from build123d import *

# Parameters (mm, degrees)
SKETCH1_W           = 49.022
SKETCH1_H           = 96.52
BOSS_EXTRUDE1_DEPTH = 7.62
SKETCH2_R           = 1.905
CUT_EXTRUDE1_DEPTH  = 55.661514075
SKETCH3_R           = 7.9375
CUT_EXTRUDE2_DEPTH  = 55.661514075
FILLET1_R           = 5.08
FILLET2_R           = 5.08
CUT_EXTRUDE3_DEPTH  = 55.661514075
SKETCH5_R           = 7.9375
SKETCH5_R_2         = 2.54
CUT_EXTRUDE4_DEPTH  = 55.661514075


with BuildPart() as part:
    # Sketch1 → Boss-Extrude1 (new body)
    with BuildSketch(Plane(origin=(0, 0, 0), x_dir=(1, 0, 0), z_dir=(0, 1, 0))):
        Rectangle(SKETCH1_W, SKETCH1_H)
    extrude(amount=BOSS_EXTRUDE1_DEPTH)

    # Sketch2 → Cut-Extrude1 (cut, through all)
    with BuildSketch(Plane(origin=(0, 7.62, 0), x_dir=(1, 0, 0), z_dir=(0, 1, 0))):
        with Locations(Location((-16.891, -44.45, 0), (0, 0, 270))):
            Circle(SKETCH2_R)
        with Locations(Location((-7.62, -44.45, 0), (0, 0, 270))):
            Circle(SKETCH2_R)
        with Locations(Location((7.62, -44.45, 0), (0, 0, 270))):
            Circle(SKETCH2_R)
        with Locations(Location((16.891, -44.45, 0), (0, 0, 270))):
            Circle(SKETCH2_R)
    extrude(amount=-CUT_EXTRUDE1_DEPTH, mode=Mode.SUBTRACT)

    # Sketch3 → Cut-Extrude2 (cut, through all)
    with BuildSketch(Plane(origin=(0, 7.62, 0), x_dir=(1, 0, 0), z_dir=(0, 1, 0))):
        with Locations(Location((0, 35.052, 0), (0, 0, 270))):
            Circle(SKETCH3_R)
    extrude(amount=-CUT_EXTRUDE2_DEPTH, mode=Mode.SUBTRACT)

    # Fillet1
    fillet1_edges = [part.edges().sort_by_distance(p)[0] for p in [
        (-24.511, 3.81, -48.26),
        (24.511, 3.81, -48.26),
    ]]
    fillet(fillet1_edges, radius=FILLET1_R)

    # Fillet2
    fillet2_edges = [part.edges().sort_by_distance(p)[0] for p in [
        (24.511, 7.62, 2.54),
        (-24.511, 7.62, 2.54),
        (0, 7.62, -48.26),
        (23.023102448, 7.62, -46.772102448),
        (-23.023102448, 7.62, -46.772102448),
    ]]
    fillet(fillet2_edges, radius=FILLET2_R)

    # Sketch4 → Cut-Extrude3 (cut, through all)
    with BuildSketch(Plane(origin=(0, 7.62, 0), x_dir=(1, 0, 0), z_dir=(0, 1, 0))):
        with BuildLine():
            Line((-1.905, -34.645821142), (-1.905, -37.185821142))
            ThreePointArc((-1.905, -37.185821142), (0, -39.090821142), (1.905, -37.185821142))
            Line((1.905, -37.185821142), (1.905, -34.645821142))
            Line((1.905, -34.645821142), (1.905, 4.217007536))
            ThreePointArc((1.905, 4.217007536), (0, 6.122007536), (-1.905, 4.217007536))
            Line((-1.905, 4.217007536), (-1.905, -34.645821142))
        make_face()
    extrude(amount=-CUT_EXTRUDE3_DEPTH, mode=Mode.SUBTRACT)

    # Sketch5 → Cut-Extrude4 (cut, through all)
    with BuildSketch(Plane(origin=(0, 7.62, 0), x_dir=(1, 0, 0), z_dir=(0, 1, 0))):
        with Locations(Location((0, 35.052, 0), (0, 0, 270))):
            Circle(SKETCH5_R)
        with Locations(Location((0, 16.002, 0), (0, 0, 270))):
            Circle(SKETCH5_R_2)
    extrude(amount=-CUT_EXTRUDE4_DEPTH, mode=Mode.SUBTRACT)


solid = part.part
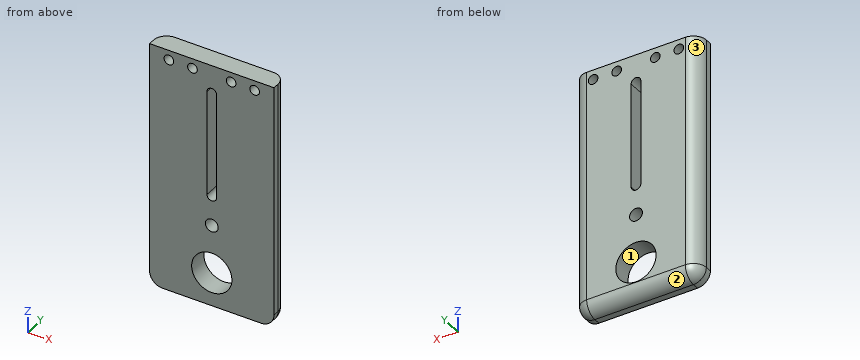
Verification items for the finished model (mm, model axes). Face numbers are marked on the shaded views. Give positions to 0.01 mm unless a question says otherwise; leave off trailing zeros. Write each loop counter-clockwise with the first axis right and the second up, starting at its lowest first coordinate (ties: lowest second). Pieces come first, ordered by that corner, then holes. Notation, with made-up numbers: M -15,-19.75 L -9,-19.75 A18 cw -9,-15.75 Z; hole C 77.5,28.25 d6. An arc over 180 degrees is marked long. Put each result on its own line as item: value. Start each with the question number.
1. Scan lines: line 1 along X through (y, z) = (3, 44.45) (3 decimals); line 2 along Z through (x, y) = (-6, 7); line 3 along Z through (x, y) = (-1.5, 6). Record each from-to range of solid material in increasing order. Write a range as [from, to].
2. Section check A-A (z = 44.45). Record the cut outline in (x, y) (3 decimals), and give its area (3 significant figures).
3. Section check D-D (y = 1.5). Give the number of separate pieces and of enclosed holes in the cut face, and give its area (3 significant figures).
4. Go/stop test with flat-tipped pins: pin 1 Ø2.5 at (y, z) = (5.5, 13) entering from -X; pin 2 Ø3 at (x, y) = (5.5, 5) entering from -Z; pin 3 Ø1.5 at (y, z) = (4.5, 28) entering from +X. Record where each tip stops, or that it passes through.
5. Section check B-B (z = 24). Record the cut outline in (x, y) (3 decimals).
6. Draft check along Z on the marked faces 1, 2 and 3. Enter one of: +Z half, -Z half, draft (parallel to the pull), parting line (faces both ways), or undercut.
7. Section check C-C (x = 0). Record the cut outline in (y, z).
Answer list:
1. line 1: [-24.49, -18.796], [-14.986, -9.525], [-5.715, 5.715], [9.525, 14.986], [18.796, 24.49]
1. line 2: [-45.61, -40.25], [-29.86, 43.45], [45.45, 48.26]
1. line 3: [-46.9, -42.85], [-27.26, -18.05], [-13.95, -5.39], [38.36, 48.26]
2. outline: M -24.511,0 L -18.796,0 L -18.796,7.62 L -19.431,7.62 A5.08 ccw -24.511,2.54 Z; M -14.986,0 L -9.525,0 L -9.525,7.62 L -14.986,7.62 Z; M -5.715,0 L 5.715,0 L 5.715,7.62 L -5.715,7.62 Z; M 9.525,0 L 14.986,0 L 14.986,7.62 L 9.525,7.62 Z; M 18.796,0 L 24.511,0 L 24.511,2.54 A5.08 ccw 19.431,7.62 L 18.796,7.62 Z
2. area: 246 mm2
3. separate pieces: 1
3. enclosed holes: 7
3. area: 4,290 mm2
4. pin 1: x = -24.21
4. pin 2: z = -48.17
4. pin 3: x = 24.36
5. outline: M -24.511,0 L -1.905,0 L -1.905,7.62 L -19.431,7.62 A5.08 ccw -24.511,2.54 Z; M 1.905,0 L 24.511,0 L 24.511,2.54 A5.08 ccw 19.431,7.62 L 1.905,7.62 Z
6. face 1: undercut
6. face 2: -Z half
6. face 3: draft
7. outline: M 0,-48.26 L 2.54,-48.26 A5.08 ccw 7.62,-43.18 L 7.62,-42.99 L 0,-42.99 Z; M 0,-27.11 L 7.62,-27.11 L 7.62,-18.54 L 0,-18.54 Z; M 0,-13.46 L 7.62,-13.46 L 7.62,-6.12 L 0,-6.12 Z; M 0,39.09 L 7.62,39.09 L 7.62,48.26 L 0,48.26 Z
